Autodesk Inventor part; units mm, degrees
ref_plane "YZ Plane" through (0, 0, 0) normal (1, 0, 0) x (0, 1, 0)
ref_plane "XZ Plane" through (0, 0, 0) normal (0, 1, 0) x (-1, 0, 0)
ref_plane "XY Plane" through (0, 0, 0) normal (0, 0, 1) x (1, 0, 0)
sketch "Sketch1" plane through (0, 0, 0) normal (0, 0, 1) x (1, 0, 0)
  line L0 (0, 0) -> (43, 0)
  line L1 (43, 0) -> (43, 43)
  line L2 (43, 43) -> (0, 43)
  line L3 (0, 43) -> (0, 0)
  dimension "d0" = 43
  dimension "d1" = 43
extrude "Extrusion1" add sketch "Sketch1" along normal blind 6.35
chamfer "Chamfer1" distance 2 angle 45 4 edges at (43, 43, 3.175) (43, 0, 3.175) (0, 43, 3.175) (0, 0, 3.175)
sketch "Sketch2" plane through (0, 0, 6.35) normal (0, 0, 1) x (1, 0, 0)
  line L0 (0, 41) -> (0, 2)
  line L1 (43, 2) -> (43, 41)
  line L2 (2, 0) -> (41, 0)
  line L3 (41, 43) -> (2, 43)
  point P0 (0, 0)
  point P1 (8, 8)
  point P2 (35, 8)
  point P3 (35, 35)
  point P4 (8, 35)
  dimension "d7" = 8
  dimension "d8" = 8
  dimension "d9" = 8
  dimension "d10" = 8
  dimension "d11" = 8
  dimension "d12" = 8
hole "Hole1" at (8, 8, 6.35) at (35, 8, 6.35) at (35, 35, 6.35) at (8, 35, 6.35) direction (0, 0, -1) diameter 3.4 depth 7 tip angle 118
ref_plane "Work Plane1" through (2, 21.5, 0) normal (0, 1, 0) x (1, 0, 0)
ref_plane "Work Plane2" through (21.5, 2, 0) normal (-1, 0, 0) x (0, 0, 1)
properties part number "Front Armor" material "Polyethylene, High Density"
Work out the finished part from the listing and answer in its coordinate system (mm). Give positions to 0.01 mm unless a question says otherwise; leave off trailing zeros. Write each loop counter-clockwise with the first axis right and the second up, starting at its lowest first coordinate (ties: lowest second). Pieces come first, ordered by that corner, then holes. Notation, with made-up numbers: (-29.75, 34) - (25.25, 34) arc R34 ccw to (25.25, 72) - close; hole circle Ø5 at (60.5, 63). An arc over 180 degrees is marked (long way). One line per item, written item: value. Start each with the question number.
1. For a pull along X with two mould halves and no side action, classify faces 1 (the flat face through (21, 22, 0)), 2 (the flat face through (42, 42, 3)), 3 (the cylindrical face through (9.03, 36.35, 3.13)) as +X half, -X half, draft (parallel to the pull), parting line (faces both ways), or undercut.
2. Find section C-C (z = 3.25). Write down the section's boundary in (x, y), then the cut area to 3 significant figures.
3. Consider probe 1 along Y at (x, z) = (8, 3.5); probe 2 along Y at (x, z) = (8.5, 1). Determine where each line is inside the solid, lowest interval first.
4. Find section A-A (y = 8). Write down the section's boundary in (x, z), then the cut area to 3 significant figures.
5. Given pin 1 (2.5 mm diameter, centred on x = 35, y = 35, fed in from -Z); pin 2 (4.5 mm diameter, centred on x = 8, y = 35, fed in from -Z), each flat-ended and moving along its own axis, determine where each tip first touches the part or whether it passes through.
Geometry results:
1. face 1: draft
1. face 2: +X half
1. face 3: undercut
2. outline: (0, 2) - (2, 0) - (41, 0) - (43, 2) - (43, 41) - (41, 43) - (2, 43) - (0, 41) - close; hole circle Ø3.4 at (8, 8); hole circle Ø3.4 at (8, 35); hole circle Ø3.4 at (35, 8); hole circle Ø3.4 at (35, 35)
2. area: 1,800 mm2
3. probe 1: 0 to 6.3, 9.7 to 33.3, 36.7 to 43
3. probe 2: 0 to 6.38, 9.62 to 33.38, 36.62 to 43
4. outline: (0, 0) - (6.3, 0) - (6.3, 6.35) - (0, 6.35) - close; (9.7, 0) - (33.3, 0) - (33.3, 6.35) - (9.7, 6.35) - close; (36.7, 0) - (43, 0) - (43, 6.35) - (36.7, 6.35) - close
4. area: 230 mm2
5. pin 1: through
5. pin 2: z = 0
